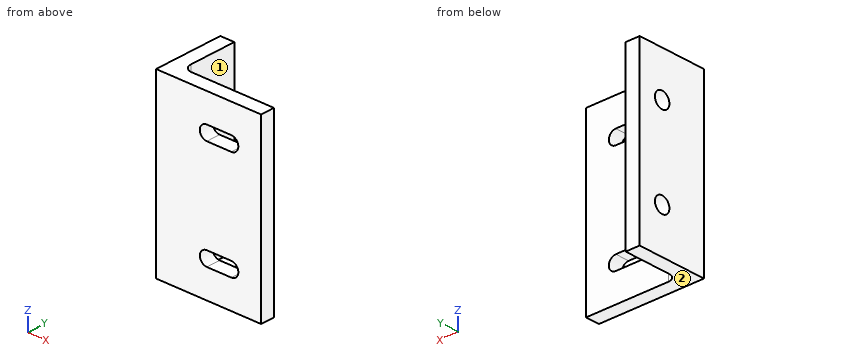
from build123d import *

# Parameters (mm, degrees)
EXTRUDE_1_DEPTH     = 100
CUT_EXTRUDE_3_DEPTH = 121.929731663
SKETCH_4_R          = 4.5
CUT_EXTRUDE_4_DEPTH = 124.288280059


with BuildPart() as part:
    # 草图1 → 凸台-拉伸1 (new body)
    with BuildSketch(Plane.XY):
        with BuildLine():
            Line((0, 0), (60, 0))
            Line((60, 0), (60, 8))
            Line((60, 8), (13, 8))
            ThreePointArc((13, 8), (9.4645, 9.4645), (8, 13))
            Line((8, 13), (8, 40))
            Line((8, 40), (0, 40))
            Line((0, 40), (0, 0))
        make_face()
    extrude(amount=EXTRUDE_1_DEPTH)

    # 草图3 → 切除-拉伸3 (cut, through all)
    with BuildSketch(Plane(origin=(0, 8, 0), x_dir=(1, 0, 0), z_dir=(0, 1, 0))):
        with BuildLine():
            Line((29, -16), (43, -16))
            ThreePointArc((43, -16), (47, -20), (43, -24))
            Line((43, -24), (29, -24))
            ThreePointArc((29, -24), (25, -20), (29, -16))
        make_face()
        with BuildLine():
            Line((29, -76), (43, -76))
            ThreePointArc((43, -76), (47, -80), (43, -84))
            Line((43, -84), (29, -84))
            ThreePointArc((29, -84), (25, -80), (29, -76))
        make_face()
    extrude(amount=-CUT_EXTRUDE_3_DEPTH, mode=Mode.SUBTRACT)

    # 草图4 → 切除-拉伸4 (cut, through all)
    with BuildSketch(Plane(origin=(0, 0, 0), x_dir=(0, 0, -1), z_dir=(1, 0, 0))):
        with Locations(Location((-25, 26, 0), (0, 0, 180))):
            Circle(SKETCH_4_R)
        with Locations(Location((-75, 26, 0), (0, 0, 180))):
            Circle(SKETCH_4_R)
    extrude(amount=CUT_EXTRUDE_4_DEPTH, mode=Mode.SUBTRACT)


solid = part.part
Can you work these out from the model? Positions are in its coordinate system, mm. Face numbers are marked on the shaded views. A direction names the side the tool comes from. Give positions to 0.01 mm unless a question says otherwise; leave off trailing zeros. Order: outer loops, then holes, each group sorted by start corner. A loop starts at its lowest first (then second) coordinate and runs counter-clockwise, first axis right, second up. Notation, with made-up numbers: M 25.5,79.25 L 77.5,79.25 A30 cw 77.5,112.25 Z; hole C -5,0.25 d1. An arc over 180 degrees is marked long. Use a Markdown table: item, result. Add a question column.
Item 1: If I drill on L1, parallel to Z at x = 3, y = 26; L2, parallel to Z at x = 32.5, y = 4; L3, parallel to Y at x = 1, z = 75, over which ranges is the centre line in solid material (lowest first)? Write a range as [from, to].
Item 2: For the marked faces 1 and 2, which set-ups out of +Z, -Z, +X, -X, +Y, -Y let a thin tool reach every point of the face, with its end or its side?
Item 3: Suppose I cut it at B-B (x = 33). List the corners of the cut face in (y, z) for me.
Item 4: Suppose I cut it at D-D (z = 64). List the corners of the cut face in (x, y) for me.
Item 5: Will these pins go through, and if not, where does the flat tip stop? pin 1 (3 mm diameter, centred on x = 39, z = 27, fed in from -Y); pin 2 (12 mm diameter, centred on y = 22.5, z = 28.5, fed in from +X); pin 3 (14 mm diameter, centred on x = 32, z = 49.5, fed in from +Y).
Item 6: Suppose I cut it at A-A (z = 25). List the corners of the cut face in (x, y) for me, then the cut area to 3 significant figures.
Item 7: Suppose I cut it at C-C (y = 26). List the corners of the cut face in (x, z) for me.
Answer sheet:
| question | item | result |
|---|---|---|
| 1 | L1 | z = [0, 20.5], [29.5, 70.5], [79.5, 100] |
| 1 | L2 | z = [0, 16], [24, 76], [84, 100] |
| 1 | L3 | y = [0, 21.5], [30.5, 40] |
| 2 | face 1 | +Z, -Z, +X, +Y |
| 2 | face 2 | -Z, +X, -X, +Y, -Y |
| 3 | outline | M 0,0 L 8,0 L 8,16 L 0,16 Z; M 0,24 L 8,24 L 8,76 L 0,76 Z; M 0,84 L 8,84 L 8,100 L 0,100 Z |
| 4 | outline | M 0,0 L 60,0 L 60,8 L 13,8 A5 cw 8,13 L 8,40 L 0,40 Z |
| 5 | pin 1 | stops at y = 0 |
| 5 | pin 2 | stops at x = 8 |
| 5 | pin 3 | stops at y = 8 |
| 6 | outline | M 0,0 L 60,0 L 60,8 L 13,8 A5 cw 8,13 L 8,21.5 L 0,21.5 Z; M 0,30.5 L 8,30.5 L 8,40 L 0,40 Z |
| 6 | area | 669 mm² |
| 7 | outline | M 0,0 L 8,0 L 8,20.5 L 0,20.5 Z; M 0,29.5 L 8,29.5 L 8,70.5 L 0,70.5 Z; M 0,79.5 L 8,79.5 L 8,100 L 0,100 Z |
